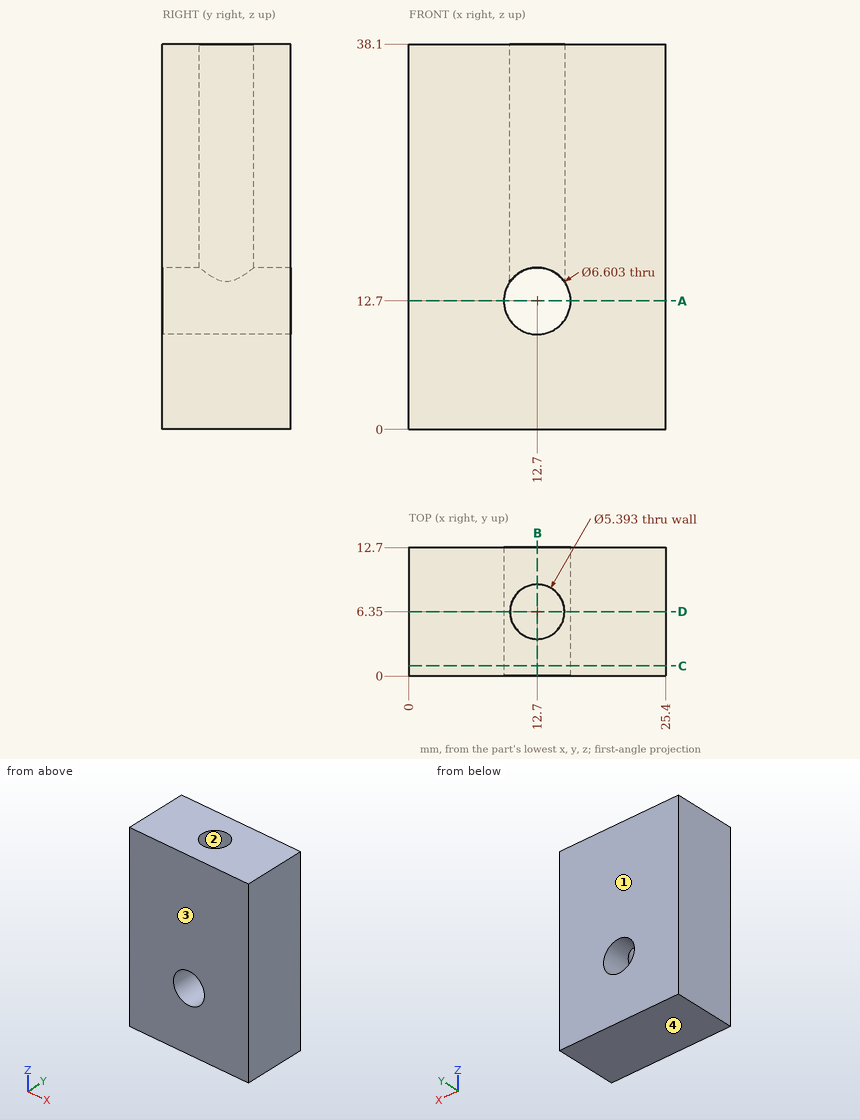
Input: dimensioned drawing with shaded views. Units: mm. Origin: part minimum x, y, z. Give positions to 0.01 mm unless a question says otherwise; leave off trailing zeros. Write each loop counter-clockwise with the first axis right and the second up, starting at its lowest first coordinate (ties: lowest second). Pieces come first, ordered by that corner, then holes. Notation, with made-up numbers: (6, 39.5) - (43, 39.5) arc R10 cw to (43, 57.5) - close; hole circle Ø9 at (70, -11). An arc over 180 degrees is marked (long way). Write item = value, one per line. Start each with the question number.
1) Cut plane C-C (y = 1). Return loops of the section in (x, z).
2) Material intervals for L1, parallel to Y at x = 12.7, z = 29.75; L2, parallel to X at y = 6.5, z = 34; L3, parallel to X at y = 8.5, z = 16 (1 decimal), sorted ascending. Write a range as [from, to].
3) Cut plane B-B (x = 12.7). Return loops of the section in (y, z).
4) Cut plane D-D (y = 6.35). Return loops of the section in (x, z) (1 decimal), and give its area (3 significant figures).
5) Cut plane A-A (z = 12.7). Return loops of the section in (x, y).
6) Draft query along Y for the marked faces 1, 2, 3 and 4. Return one class per face: pulls with the +Y half, pulls with the -Y half, needs draft (parallel to the pull), parting line crosses it, or undercut.
Answers follow:
q1.outline = (0, 0) - (25.4, 0) - (25.4, 38.1) - (0, 38.1) - close; hole circle Ø6.6 at (12.7, 12.7)
q2.L1 = [0, 3.65], [9.05, 12.7]
q2.L2 = [0, 10.01], [15.39, 25.4]
q2.L3 = [0, 11.1], [14.3, 25.4]
q3.outline = (0, 0) - (12.7, 0) - (12.7, 9.4) - (0, 9.4) - close; (0, 16) - (3.65, 16) - (3.65, 38.1) - (0, 38.1) - close; (9.05, 16) - (12.7, 16) - (12.7, 38.1) - (9.05, 38.1) - close
q4.outline = (0, 0) - (25.4, 0) - (25.4, 38.1) - (15.4, 38.1) - (15.4, 14.6) arc R3.3 cw (long way) to (10, 14.6) - (10, 38.1) - (0, 38.1) - close
q4.area = 812 mm^2
q5.outline = (0, 0) - (9.4, 0) - (9.4, 12.7) - (0, 12.7) - close; (16, 0) - (25.4, 0) - (25.4, 12.7) - (16, 12.7) - close
q6.face_1 = pulls with the +Y half
q6.face_2 = undercut
q6.face_3 = pulls with the -Y half
q6.face_4 = needs draft
